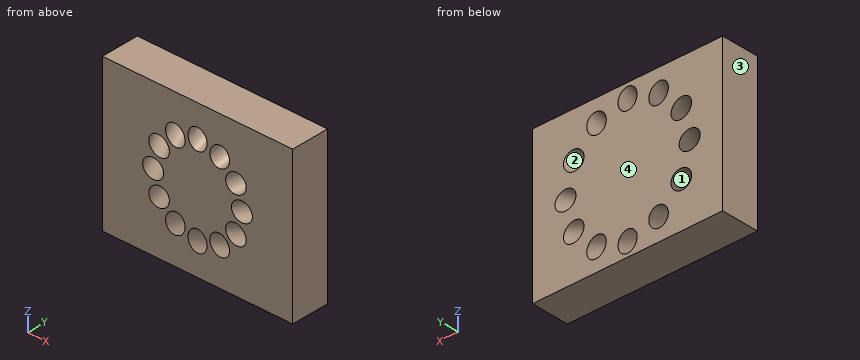
```python
from build123d import *

# Parameters (mm, degrees)
SKIZZE1_W                       = 100
SKIZZE1_H                       = 80
AUFSATZ_LINEAR_AUSTRAGEN1_DEPTH = 20
KREISMUSTER1_COUNT              = 12


with BuildPart() as part:
    # Skizze1 → Aufsatz-Linear austragen1 (new body)
    with BuildSketch(Plane(origin=(0, 0, 0), x_dir=(1, 0, 0), z_dir=(0, 1, 0))):
        Rectangle(SKIZZE1_W, SKIZZE1_H)
    extrude(amount=AUFSATZ_LINEAR_AUSTRAGEN1_DEPTH)

    # Skizze2 → Schnitt-Rotation1 (revolve, cut)
    with BuildSketch(Plane.XY):
        Polygon((-33.62688673, 22.113091309), (-22.330032248, -2.113091309), (-17.798493313, 0), (-29.095347795, 24.226182617), align=None)
    schnitt_rotation1 = revolve(axis=Axis((0, -50, 0), (-0.422618262, 0.906307787, 0)), mode=Mode.SUBTRACT)

    # Kreismuster1: Schnitt-Rotation1 ×12 about axis
    kreismuster1_axis = Axis((0, 0, 0), (0, 1, 0))
    for i in range(1, KREISMUSTER1_COUNT):
        add(schnitt_rotation1.rotate(kreismuster1_axis, i * 360 / KREISMUSTER1_COUNT), mode=Mode.SUBTRACT)


solid = part.part
```
Work out the finished part from the listing and answer in its coordinate system (mm). Face numbers are marked on the shaded views. Coordinates: 2 decimals unless noted, no trailing zeros.
Q1. Find the intervals of material crossed by line 1 (Z direction, x = 28.5, y = 16.5); line 2 (X direction, y = 9.5, z = -16.5); line 3 (Z direction, x = -16, y = 18.75), in increasing order.
Q2. Determine the mould class of the marked faces 1, 2, 3 and 4 for opening direction Y: released by +Y, released by -Y, zero draft, split by the parting line, or undercut.
Q3. This flat-tipped pin is pushed along its axis until it touches: pin 1 Ø5 at (x, z) = (2, 0) entering from -Y. Where does it stop, or does it pass through?
Q4. A cutting plane is placed at A-A, the plane y = 1.5. State how many separate pieces and enclosed holes the cut face has, then the cut area to 3 significant figures.
Findings below:
1. line 1: z = -40 to -20.51, -10.77 to -4.45, 4.45 to 10.77, 20.51 to 40
1. line 2: x = -50 to -28.88, -19.65 to 19.65, 28.88 to 50
1. line 3: z = -40 to -33.13, -22.39 to 22.39, 33.13 to 40
2. face 1: undercut
2. face 2: undercut
2. face 3: zero draft
2. face 4: released by +Y
3. pin 1: stops at y = 0
4. separate pieces: 1
4. enclosed holes: 12
4. area: 6,960 mm2
